from build123d import *

# Parameters (mm, degrees)
SKETCH_W        = 36
SKETCH_H        = 50
PAD_DEPTH       = 8
PAD001_DEPTH    = 13
SKETCH004_W     = 11
SKETCH004_H     = 4
PAD003_DEPTH    = 13
PAD002_DEPTH    = 13
SKETCH005_W     = 25.977524
SKETCH005_H     = 13
POCKET_DEPTH    = 5
SKETCH006_R     = 1.5
POCKET001_DEPTH = 5
SKETCH007_R     = 1.5
POCKET002_DEPTH = 5
CHAMFER_SIZE    = 2
CHAMFER001_SIZE = 2
CHAMFER002_SIZE = 3
CHAMFER003_SIZE = 2
SKETCH008_W     = 23.210894
SKETCH008_H     = 13
POCKET003_DEPTH = 2
CHAMFER004_SIZE = 1
SKETCH009_W     = 14.868066
SKETCH009_H     = 8
PAD004_DEPTH    = 2
FILLET_R        = 1
FILLET001_R     = 1
FILLET002_R     = 1
SKETCH011_W     = 14.090648
SKETCH011_H     = 8
PAD005_DEPTH    = 5
FILLET003_R     = 1
SKETCH012_R     = 1.5
POCKET004_DEPTH = 8.001
SKETCH013_R     = 2.75
POCKET005_DEPTH = 3
SKETCH014_W     = 18.80099
SKETCH014_H     = 2
POCKET006_DEPTH = 7


with BuildPart() as pad003:
    # Sketch → Pad (new body)
    with BuildSketch(Plane.XY):
        Rectangle(SKETCH_W, SKETCH_H)
    extrude(amount=PAD_DEPTH)

    # Sketch002 → Pad001 (new body)
    with BuildSketch(Plane.XY.offset(8)):
        Polygon((-13.5, -25), (13.5, -25), (13.5, -19.629501), (11.5, -19.629501), (11.5, -23), (-11.5, -23), (-11.5, -18.969727), (-13.5, -18.969727), align=None)
    extrude(amount=PAD001_DEPTH)

    # Sketch004 → Pad003 (new body)
    with BuildSketch(Plane.XY.offset(8)):
        with Locations((4.8652, 22.5)):
            Rectangle(SKETCH004_W, SKETCH004_H)
    extrude(amount=PAD003_DEPTH)


with BuildPart() as pocket006:
    # Sketch003 → Pad002 (new body)
    with BuildSketch(Plane.XY.offset(8)):
        Polygon((11.3, 2), (18, 2), (18, -5), (16.3, -5), (16.3, -2), (11.3, -2), align=None)
        Polygon((-11.3, 2), (-18, 2), (-18, -5), (-16.3, -5), (-16.3, -2), (-11.3, -2), align=None)
    extrude(amount=PAD002_DEPTH)

    # Fusion: union Pad003
    add(pad003.part)

    # Sketch005 → Pocket (cut)
    with BuildSketch(Plane.XY.offset(8)):
        with Locations((5.011238, 13.5)):
            Rectangle(SKETCH005_W, SKETCH005_H)
    extrude(amount=-POCKET_DEPTH, mode=Mode.SUBTRACT)

    # Sketch006 → Pocket001 (cut)
    with BuildSketch(Plane(origin=(0, 2, 0), x_dir=(-1, 0, 0), z_dir=(0, 1, 0))):
        with Locations((-14.3, 13.9)):
            Circle(SKETCH006_R)
        with Locations((14.3, 13.9)):
            Circle(SKETCH006_R)
    extrude(amount=-POCKET001_DEPTH, mode=Mode.SUBTRACT)

    # Sketch007 → Pocket002 (cut)
    with BuildSketch(Plane(origin=(0, 24.5, 0), x_dir=(-1, 0, 0), z_dir=(0, 1, 0))):
        with Locations((-4.854515, 13.9)):
            Circle(SKETCH007_R)
    extrude(amount=-POCKET002_DEPTH, mode=Mode.SUBTRACT)

    # Chamfer
    chamfer_edges = [pocket006.edges().sort_by_distance(p)[0] for p in [
        (18, 13.5, 3),
    ]]
    chamfer(chamfer_edges, length=CHAMFER_SIZE)

    # Chamfer001
    chamfer001_edges = [pocket006.edges().sort_by_distance(p)[0] for p in [
        (16, 13.5, 3),
    ]]
    chamfer(chamfer001_edges, length=CHAMFER001_SIZE)

    # Chamfer002
    chamfer002_edges = [pocket006.edges().sort_by_distance(p)[0] for p in [
        (14, 13.5, 3),
    ]]
    chamfer(chamfer002_edges, length=CHAMFER002_SIZE)

    # Chamfer003
    chamfer003_edges = [pocket006.edges().sort_by_distance(p)[0] for p in [
        (11, 13.5, 3),
    ]]
    chamfer(chamfer003_edges, length=CHAMFER003_SIZE)

    # Sketch008 → Pocket003 (cut)
    with BuildSketch(Plane.XY.offset(3)):
        with Locations((7.17125, 13.5)):
            Rectangle(SKETCH008_W, SKETCH008_H)
    extrude(amount=-POCKET003_DEPTH, mode=Mode.SUBTRACT)

    # Chamfer004
    chamfer004_edges = [pocket006.edges().sort_by_distance(p)[0] for p in [
        (-4.434197, 13.5, 3),
    ]]
    chamfer(chamfer004_edges, length=CHAMFER004_SIZE)

    # Sketch009 → Pad004 (new body)
    with BuildSketch(Plane.YZ.offset(18)):
        with Locations((-12.37453, 4)):
            Rectangle(SKETCH009_W, SKETCH009_H)
    extrude(amount=PAD004_DEPTH)

    # Fillet
    fillet_edges = [pocket006.edges().sort_by_distance(p)[0] for p in [
        (20, -19.808563, 4),
        (20, -4.940497, 4),
    ]]
    fillet(fillet_edges, radius=FILLET_R)

    # Fillet001
    fillet001_edges = [pocket006.edges().sort_by_distance(p)[0] for p in [
        (18, -25, 4),
        (18, 25, 4),
    ]]
    fillet(fillet001_edges, radius=FILLET001_R)

    # Fillet002
    fillet002_edges = [pocket006.edges().sort_by_distance(p)[0] for p in [
        (-18, 25, 4),
        (-18, -25, 4),
    ]]
    fillet(fillet002_edges, radius=FILLET002_R)

    # Sketch011 → Pad005 (new body)
    with BuildSketch(Plane(origin=(-18, 0, 0), x_dir=(0, -1, 0), z_dir=(-1, 0, 0))):
        with Locations((12.277352, 4)):
            Rectangle(SKETCH011_W, SKETCH011_H)
    extrude(amount=PAD005_DEPTH)

    # Fillet003
    fillet003_edges = [pocket006.edges().sort_by_distance(p)[0] for p in [
        (-23, -5.232028, 4),
        (-23, -19.322676, 4),
    ]]
    fillet(fillet003_edges, radius=FILLET003_R)

    # Sketch012 → Pocket004 (cut, through all)
    with BuildSketch(Plane.XY.offset(8)):
        with Locations((-17.58419, -12.3304)):
            Circle(SKETCH012_R)
        with Locations((15.481561, -12.3304)):
            Circle(SKETCH012_R)
        with Locations((-12.798991, 19.810022)):
            Circle(SKETCH012_R)
    extrude(amount=-POCKET004_DEPTH, mode=Mode.SUBTRACT)

    # Sketch013 → Pocket005 (cut)
    with BuildSketch(Plane.XY.offset(8)):
        with Locations((-17.584191, -12.2855)):
            Circle(SKETCH013_R)
        with Locations((15.465243, -12.2855)):
            Circle(SKETCH013_R)
        with Locations((-12.792856, 19.795126)):
            Circle(SKETCH013_R)
    extrude(amount=-POCKET005_DEPTH, mode=Mode.SUBTRACT)

    # Sketch014 → Pocket006 (cut)
    with BuildSketch(Plane.XY.offset(8)):
        with Locations((5.024045, 6)):
            Rectangle(SKETCH014_W, SKETCH014_H)
    extrude(amount=-POCKET006_DEPTH, mode=Mode.SUBTRACT)


solid = pocket006.part
Part model, mm, in its own coordinate system. A direction names the side the tool comes from. Give positions to 0.01 mm unless a question says otherwise; leave off trailing zeros. Order: outer loops, then holes, each group sorted by start corner. A loop starts at its lowest first (then second) coordinate and runs counter-clockwise, first axis right, second up. Notation, with made-up numbers: (82.5, 39.5) - (126.5, 39.5) arc R13 ccw to (126.5, 54.5) - close; hole circle Ø11 at (70.25, -20.75). An arc over 180 degrees is marked (long way). Use a Markdown table: item, result.
1) Saw through at D-D on x = 2. List the corners of the cut face in (y, z).
Checked values:
| item | result |
|---|---|
| outline | (-25, 0) - (25, 0) - (25, 8) - (24.5, 8) - (24.5, 21) - (20.5, 21) - (20.5, 8) - (20, 8) - (20, 1) - (5, 1) - (5, 8) - (-23, 8) - (-23, 21) - (-25, 21) - close |
2) Saw through at B-B on x = 15. List the corners of the cut face in (y, z).
Checked values:
| item | result |
|---|---|
| outline | (-25, 0) - (-13.75, 0) - (-13.75, 5) - (-15, 5) - (-15, 8) - (-25, 8) - close; (-10.91, 0) - (25, 0) - (25, 8) - (20, 8) - (20, 1) - (7, 1) - (7, 8) - (2, 8) - (2, 12.57) - (-2, 12.57) - (-2, 8) - (-9.58, 8) - (-9.58, 5) - (-10.91, 5) - close; (-2, 15.23) - (2, 15.23) - (2, 21) - (-2, 21) - close |
3) Flat gauge pins, fed straight in: P1, Ø2.5, axis at x = 4.85, z = 13.9, coming from the +Y side; P2, Ø6.5, axis at y = -23.5, z = 13, coming from the -X side; P3, Ø0.5, axis at x = 18.5, z = 4.5, coming from the -Y side. Where does each tip first touch, or does it go through?
Checked values:
| item | result |
|---|---|
| P1 | y = -23 |
| P2 | x = -13.5 |
| P3 | y = -19.81 |
4) Saw through at A-A on z = 18.5. List the corners of the cut face in (x, y).
Checked values:
| item | result |
|---|---|
| outline | (-18, -5) - (-16.3, -5) - (-16.3, -2) - (-11.3, -2) - (-11.3, 2) - (-18, 2) - close; (-13.5, -25) - (13.5, -25) - (13.5, -19.63) - (11.5, -19.63) - (11.5, -23) - (-11.5, -23) - (-11.5, -18.97) - (-13.5, -18.97) - close; (-0.63, 20.5) - (10.37, 20.5) - (10.37, 24.5) - (-0.63, 24.5) - close; (11.3, -2) - (16.3, -2) - (16.3, -5) - (18, -5) - (18, 2) - (11.3, 2) - close |
5) Probe L1, parallel to Y at x = -3.5, z = 3.25; L2, parallel to X at y = -12.5, z = 6.5; L3, parallel to X at y = -2.5, z = 15.5. List the from-to ranges inside material, lowest first. Write a range as from..to.
Checked values:
| item | result |
|---|---|
| L1 | -25..5, 20..25 |
| L2 | -23..-20.33, -14.84..12.72, 18.21..20 |
| L3 | -18..-16.3, 16.3..18 |
6) 3-axis set-ups, long thin cutter, end or side, ignore diameter. For faces 1 (the flat face through (-16.3, -4, 14)), 2 (the flat face through (-7, 14, 3)), 3 (the flat face through (-20, -5.232, 4)), 4 (the flat face through (12.7, -2, 14.4)): which of +Z, -Z, +X, -X, +Y, -Y reach the whole face in a straight line?
Checked values:
| item | result |
|---|---|
| face 1 | +Z, -Y |
| face 2 | +Z, +X |
| face 3 | +Z, -Z, -X, +Y |
| face 4 | +Z |
7) Saw through at C-C on z = 6.25. Count the separate pieces of the cut face and the enclosed holes in it, plus the area to 3 significant figures.
Checked values:
| item | result |
|---|---|
| separate pieces | 1 |
| enclosed holes | 3 |
| area | 1,450 mm² |
